Source: CAD feature listing. Evaluate the final solid. Frame: model axes, mm. A direction names the side the tool comes from. Coordinates: 2 decimals unless noted, no trailing zeros. Loops run counter-clockwise (first coordinate to the right, second up) from the corner with the lowest first, then second, coordinate; pieces in that order, holes last. Notation, with made-up numbers: (-35.5, 51.5) - (-16.5, 51.5) arc R11 cw to (-16.5, 66.5) - close; hole circle Ø9 at (82, 58.5). An arc over 180 degrees is marked (long way). Write item = value, one per line. Start each with the question number.
Autodesk Inventor part; units mm, degrees
ref_plane "YZ Plane" through (0, 0, 0) normal (1, 0, 0) x (0, 1, 0)
ref_plane "XZ Plane" through (0, 0, 0) normal (0, 1, 0) x (-1, 0, 0)
ref_plane "XY Plane" through (0, 0, 0) normal (0, 0, 1) x (1, 0, 0)
sketch "Sketch1" plane through (0, 0, 0) normal (0, 0, 1) x (1, 0, 0)
  line L0 (9.2486, 13.3739) -> (9.2486, 48.3739)
  line L1 (9.2486, 13.3739) -> (69.2486, 13.3739)
  line L2 (69.2486, 13.3739) -> (69.2486, 43.3739)
  line L3 (69.2486, 43.3739) -> (9.2486, 48.3739)
  line L4 (69.2486, 63.4432) -> (9.2486, 68.4432)
  line L5 (9.2486, 48.3739) -> (9.2486, 68.4432)
  line L6 (69.2486, 43.3739) -> (69.2486, 63.4432)
  point P0 (0, 0)
  dimension "d0" = 35
  dimension "d1" = 60
  dimension "d2" = 30
  dimension "d3" = 20
extrude "Extrusion1" add sketch "Sketch1" along normal blind 45 and the other way blind 5 contours L0 L3 L2 L1
extrude "Extrusion2" add sketch "Sketch1" against normal blind 5 contours L5 L4 L6 L3
extrude "Extrusion3" add sketch "Sketch1" along normal blind 45 contours L5 L4 L6 L3
extrude "Extrusion4" cut sketch "Sketch1" along normal blind 40 contours L5 L4 L6 L3
properties part number "collectionslideintoscrew"
Item 1: Cut plane C-C (z = 12). Return the cut outline in (x, y).
Item 2: Reachability of faces 1 (the flat face through (39.67, 65.91, 42.46)), 2 (the flat face through (39, 56, 0)) from +Z, -Z, +X, -X, +Y, -Y: full face, straight path, thin tool, end or side. Return the list, or none.
Item 3: Cut plane A-A (y = 57). Return the cut outline in (x, z), then the cut area to 3 significant figures.
Item 4: Cut plane B-B (x = 38). Return the cut outline in (y, z).
Item 5: Cut plane D-D (y = 45.5). Return the cut outline in (x, z).
Item 6: Material intervals for L1, parallel to Z at x = 34, y = 51; L2, parallel to Y at x = 12.5, z = -1; L3, parallel to Y at x = 61.5, z = 35.5, sorted ascending. Write a range as [from, to].
Item 7: Draft query along Z for faces 3 (the flat face through (39.67, 65.91, -2.54)), 4 (the flat face through (39, 41, 45)), 5 (the flat face through (39, 56, 40)). Return one class per face: released by +Z, released by -Z, zero draft, split by the parting line, or undercut.
Responses:
q1.outline = (9.25, 13.37) - (69.25, 13.37) - (69.25, 43.37) - (9.25, 48.37) - close
q2.face_1 = +Z, -Z, +X, +Y
q2.face_2 = +X, +Y
q3.outline = (9.25, -5) - (69.25, -5) - (69.25, 0) - (9.25, 0) - close; (9.25, 40) - (69.25, 40) - (69.25, 45) - (9.25, 45) - close
q3.area = 600 mm2
q4.outline = (13.37, -5) - (66.05, -5) - (66.05, 0) - (45.98, 0) - (45.98, 40) - (66.05, 40) - (66.05, 45) - (13.37, 45) - close
q5.outline = (9.25, -5) - (69.25, -5) - (69.25, 0) - (43.74, 0) - (43.74, 40) - (69.25, 40) - (69.25, 45) - (9.25, 45) - close
q6.L1 = [-5, 0], [40, 45]
q6.L2 = [13.37, 68.17]
q6.L3 = [13.37, 44.02]
q7.face_3 = zero draft
q7.face_4 = released by +Z
q7.face_5 = undercut
